Autodesk Inventor part; units mm, degrees
ref_plane "YZ Plane" through (0, 0, 0) normal (1, 0, 0) x (0, 1, 0)
ref_plane "XZ Plane" through (0, 0, 0) normal (0, 1, 0) x (-1, 0, 0)
ref_plane "XY Plane" through (0, 0, 0) normal (0, 0, 1) x (1, 0, 0)
sketch "Sketch1" plane through (0, 0, 0) normal (0, 0, 1) x (1, 0, 0)
  line L0 (0, 0) -> (22, 0)
  line L1 (22, 0) -> (22, 10)
  line L2 (0, 0) -> (0, 10)
  line L3 (8.5, 15) -> (13.5, 15)
  line L4 (13.5, 15) -> (22, 10)
  line L5 (8.5, 15) -> (0, 10)
  dimension "d0" = 22
  dimension "d1" = 10
  dimension "d2" = 5
  dimension "d3" = 5
extrude "Extrusion1" add sketch "Sketch1" along normal blind 8.5
sketch "Sketch2" plane through (0, 0, 8.5) normal (0, 0, 1) x (1, 0, 0)
  line L0 (0, 0) -> (22, 0)
  line L1 (22, 0) -> (22, 10)
  line L2 (13.5, 15) -> (8.5, 15)
  arc A0 (10, 8.873) -> (12, 8.873) centre (11, 5) ccw
  circle A1 centre (11, 5) radius 2.1
  line L3 (10, 15) -> (10, 8.873)
  line L4 (12, 8.873) -> (12, 15)
  dimension "d6" = 8
  dimension "d7" = 4.2
  dimension "d8" = 5
  dimension "d9" = 11
  dimension "d10" = 2
  dimension "d11" = 1
extrude "Extrusion2" cut sketch "Sketch2" against normal blind 7.5
fillet "Fillet1" radius 3 2 edges at (12, 8.873, 4.75) (10, 8.873, 4.75)
sketch "Sketch3" plane through (8.5, 15, 0) normal (0, 1, 0) x (1, 0, 0)
  line L0 (13.5, 0) -> (5, 0)
  line L1 (5, 0) -> (5, -8.5)
  line L2 (13.5, -8.5) -> (5, -8.5)
  line L3 (13.5, 0) -> (13.5, -8.5)
  line L4 (0, 0) -> (-8.5, 0)
  line L5 (-8.5, 0) -> (-8.5, -8.5)
  line L6 (0, -8.5) -> (-8.5, -8.5)
  line L7 (0, 0) -> (0, -8.5)
  point P0 (9.25, -4.25)
  point P1 (-4.25, -4.25)
  dimension "d15" = 13.5
  dimension "d16" = 4.25
  dimension "d17" = 4.25
hole "Hole1" at (17.75, 15, 4.25) at (4.25, 15, 4.25) direction (0, -1, 0) diameter 3.5 end through all counterbore diameter 8 counterbore depth 5
properties part number "XCarriageBeltClipRound"
The model under review builds one solid part; all positions refer to its coordinate system, in mm. A direction names the side the tool comes from. Round coordinates to 2 decimals unless told otherwise and drop trailing zeros. Loops run counter-clockwise (first coordinate to the right, second up) from the corner with the lowest first, then second, coordinate; pieces in that order, holes last. Notation, with made-up numbers: (88.25, 55) - (110.25, 55) arc R20 cw to (110.25, 63) - close; hole circle Ø9 at (56.5, -21.5). An arc over 180 degrees is marked (long way). Use a Markdown table: item, result. Add a question column.
Q1. Add section C-C (y = 5). State the section outline as (x, z) points, plus the area to 3 significant figures.
Q2. Insertion check: pin 1 Ø3 at (y, z) = (9, 1.5) entering from -X; pin 2 Ø5 at (x, z) = (17.75, 4.25) entering from +Y; pin 3 Ø3 at (x, z) = (17.75, 4.25) entering from +Y; pin 4 Ø2 at (y, z) = (13.5, 6) entering from +X. Each pin has a flat end and moves straight along its axis. Give the tip position at first contact, or say it passes through.
Q3. Machinability: for faces 5 (the face through (19.5, 10, 5.1)), 6 (the face through (9.85, 15, 4.19)), 7 (the face through (12.35, 9.34, 4.7)), 8 (the face through (10, 13, 5)), which of the approach directions +Z, -Z, +X, -X, +Y, -Y give a long, thin tool a straight path to every point of the face, cutting with its end or side? Answer none if there is none.
Q4. Add section B-B (z = 5). State how many separate pieces and enclosed holes the cut face has, plus the area to 3 significant figures.
Q5. Add section A-A (x = 4.25). State the section outline as (y, z) points, plus the area to 4 significant figures.
Q6. The part is to be moulded in two halves that separate along X. For faces 1 (the face through (11, 0, 4)), 2 (the face through (8.155, 11.856, 3.383)), 3 (the face through (12, 13, 5)), 4 (the face through (22, 5, 4)), say which applies: pulls with the +X half, pulls with the -X half, needs draft (parallel to the pull), parting line crosses it, or undercut.
Q7. For probe 1 along Y at (x, z) = (11, 6.75); probe 2 along X at (y, z) = (6.25, 4.25); probe 3 along Z at (x, y) = (4.25, 2.5), list the stretches that pass through material, from the lowest coordinate up.
Q8. Add section D-D (z = 2). State the section outline as (x, y) points.
Worked answers:
| question | item | result |
|---|---|---|
| 1 | outline | (0, 0) - (22, 0) - (22, 8.5) - (15, 8.5) - (15, 1) - (13.1, 1) - (13.1, 8.5) - (8.9, 8.5) - (8.9, 1) - (7, 1) - (7, 8.5) - (0, 8.5) - close; hole circle Ø3.5 at (4.25, 4.25); hole circle Ø3.5 at (17.75, 4.25) |
| 1 | area | 139 mm² |
| 2 | pin 1 | x = 0 |
| 2 | pin 2 | y = 10 |
| 2 | pin 3 | through |
| 2 | pin 4 | x = 14.85 |
| 3 | face 5 | +Y |
| 3 | face 6 | +Z, -Z, +X, -X, +Y |
| 3 | face 7 | +Z |
| 3 | face 8 | +Z, +Y |
| 4 | separate pieces | 4 |
| 4 | enclosed holes | 0 |
| 4 | area | 135 mm² |
| 5 | outline | (0, 0) - (12.5, 0) - (12.5, 0.25) - (10, 0.25) - (10, 2.5) - (0, 2.5) - close; (0, 6) - (10, 6) - (10, 8.25) - (12.5, 8.25) - (12.5, 8.5) - (0, 8.5) - close |
| 5 | area | 51.25 mm² |
| 6 | face 1 | needs draft |
| 6 | face 2 | undercut |
| 6 | face 3 | undercut |
| 6 | face 4 | pulls with the +X half |
| 7 | probe 1 | 0 to 1, 2.9 to 7.1 |
| 7 | probe 2 | 0 to 2.5, 6 to 7.2, 9.31 to 12.69, 14.8 to 16, 19.5 to 22 |
| 7 | probe 3 | 0 to 2.5, 6 to 8.5 |
| 8 | outline | (0, 0) - (22, 0) - (22, 10) - (21.06, 10.55) - (21.06, 10) - (14.44, 10) - (14.44, 14.45) - (13.5, 15) - (12, 15) - (12, 10.74) arc R3 ccw to (13.29, 8.28) arc R4 cw (long way) to (8.71, 8.28) arc R3 ccw to (10, 10.74) - (10, 15) - (8.5, 15) - (7.56, 14.45) - (7.56, 10) - (0.94, 10) - (0.94, 10.55) - (0, 10) - close; circle Ø4.2 at (11, 5) |
